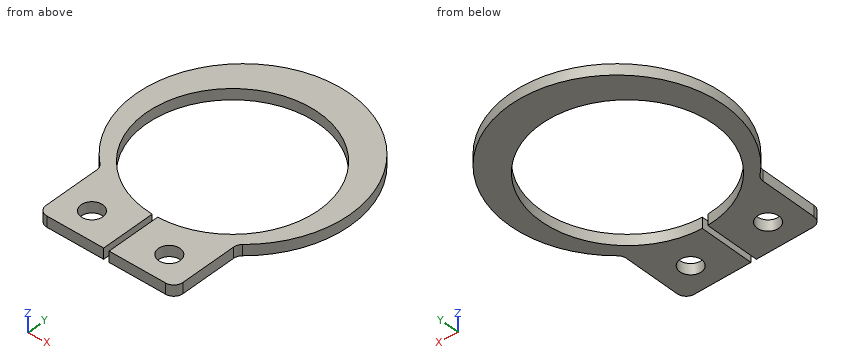
```python
from build123d import *

# Parameters (mm, degrees)
BOSS_EXTRUDE1_DEPTH = 0.6
SKETCH2_R           = 0.6
CUT_EXTRUDE1_DEPTH  = 1.6


with BuildPart() as part:
    # Sketch1 → Boss-Extrude1 (new body)
    with BuildSketch(Plane.XY):
        with BuildLine():
            Line((-3.8, -4.157546152), (-3.8, -7.3))
            ThreePointArc((-3.8, -7.3), (-3.653553391, -7.653553391), (-3.3, -7.8))
            Line((-3.3, -7.8), (-0.15, -7.8))
            Line((-0.15, -7.8), (-0.15, -4.797655678))
            ThreePointArc((-0.15, -4.797655678), (0, 4.8), (0.15, -4.797655678))
            Line((0.15, -4.797655678), (0.15, -7.8))
            Line((0.15, -7.8), (3.3, -7.8))
            ThreePointArc((3.3, -7.8), (3.653553391, -7.653553391), (3.8, -7.3))
            Line((3.8, -7.3), (3.8, -4.157546152))
            ThreePointArc((3.8, -4.157546152), (3.843564535, -3.953422006), (3.966666667, -3.784868155))
            ThreePointArc((3.966666667, -3.784868155), (0, 6.6), (-3.966666667, -3.784868155))
            ThreePointArc((-3.966666667, -3.784868155), (-3.843564535, -3.953422006), (-3.8, -4.157546152))
        make_face()
    extrude(amount=-BOSS_EXTRUDE1_DEPTH)

    # Sketch2 → Cut-Extrude1 (cut, through all)
    with BuildSketch(Plane.XY):
        with Locations((-2.15, -6.3)):
            Circle(SKETCH2_R)
        with Locations((2.15, -6.3)):
            Circle(SKETCH2_R)
    extrude(amount=-CUT_EXTRUDE1_DEPTH, mode=Mode.SUBTRACT)


solid = part.part
```
Work out the finished part from the listing and answer in its coordinate system (mm). Give positions to 0.01 mm unless a question says otherwise; leave off trailing zeros. Write each loop counter-clockwise with the first axis right and the second up, starting at its lowest first coordinate (ties: lowest second). Pieces come first, ordered by that corner, then holes.
(1) The part is cut by section B-B on z = -0.5. Write down the section's boundary in (x, y), plus the area to 3 significant figures.
Final values:
outline: (-3.97, -3.78) arc R0.5 cw to (-3.8, -4.16) - (-3.8, -7.3) arc R0.5 ccw to (-3.3, -7.8) - (-0.15, -7.8) - (-0.15, -4.8) arc R4.8 cw (long way) to (0.15, -4.8) - (0.15, -7.8) - (3.3, -7.8) arc R0.5 ccw to (3.8, -7.3) - (3.8, -4.16) arc R0.5 cw to (3.97, -3.78) arc R5.95 ccw (long way) to start; hole circle Ø1.2 at (-2.15, -6.3); hole circle Ø1.2 at (2.15, -6.3)
area: 57.9 mm2
(2) Straight lines are drawn through the part: line 1 (X direction, y = -6, z = -0.4); line 2 (X direction, y = -7, z = -0.2); line 3 (Y direction, x = 2.15, z = -0.4). For each, find the intervals that lie inside material, in ascending order.
Final values:
line 1: x = -3.8 to -2.67, -1.63 to -0.15, 0.15 to 1.63, 2.67 to 3.8
line 2: x = -3.8 to -0.15, 0.15 to 3.8
line 3: y = -7.8 to -6.9, -5.7 to -4.29, 4.29 to 6.2
(3) The part is cut by section C-C on x = -3. Write down the section's boundary in (y, z).
Final values:
outline: (-7.8, -0.6) - (-3.75, -0.6) - (-3.75, 0) - (-7.8, 0) - close; (3.75, -0.6) - (5.79, -0.6) - (5.79, 0) - (3.75, 0) - close
(4) Flat-ended cylindrical pins translate along their axes: pin 1 Ø1 at (x, y) = (2.15, -6.3) entering from -Z; pin 2 Ø4 at (x, y) = (0.5, 3) entering from -Z. Find the tip coordinate at first contact, or state that the pin passes through.
Final values:
pin 1: passes through
pin 2: stops at z = -0.6
(5) The part is cut by section A-A on y = -6.3. Write down the section's boundary in (x, z).
Final values:
outline: (-3.8, -0.6) - (-2.75, -0.6) - (-2.75, 0) - (-3.8, 0) - close; (-1.55, -0.6) - (-0.15, -0.6) - (-0.15, 0) - (-1.55, 0) - close; (0.15, -0.6) - (1.55, -0.6) - (1.55, 0) - (0.15, 0) - close; (2.75, -0.6) - (3.8, -0.6) - (3.8, 0) - (2.75, 0) - close
(6) The part is cut by section D-D on y = 2.5. Write down the section's boundary in (x, z), plus the area to 3 significant figures.
Final values:
outline: (-5.66, -0.6) - (-4.1, -0.6) - (-4.1, 0) - (-5.66, 0) - close; (4.1, -0.6) - (5.66, -0.6) - (5.66, 0) - (4.1, 0) - close
area: 1.87 mm2
